from build123d import *

# Parameters (mm, degrees)
F0_R     = 2.867556
F1_DEPTH = 20
F3_DEPTH = 5


with BuildPart() as f1:
    # F0 (on Top) → F1 (new body)
    with BuildSketch(Plane.XY):
        Polygon((49.845867, -3.922955), (45, 0), (49.845867, 3.922955), (44.445975, 7.039551), (48.618496, 11.672268), (42.797543, 13.905765), (46.193977, 19.134172), (40.095294, 20.429572), (42.632008, 26.124928), (36.405765, 26.450336), (38.020298, 32.472402), (31.819805, 31.819805), (32.472402, 38.020298), (26.450336, 36.405765), (26.124928, 42.632008), (20.429572, 40.095294), (19.134172, 46.193977), (13.905765, 42.797543), (11.672268, 48.618496), (7.039551, 44.445975), (3.922955, 49.845867), (0, 45), (-3.922955, 49.845867), (-7.039551, 44.445975), (-11.672268, 48.618496), (-13.905765, 42.797543), (-19.134172, 46.193977), (-20.429572, 40.095294), (-26.124928, 42.632008), (-26.450336, 36.405765), (-32.472402, 38.020298), (-31.819805, 31.819805), (-38.020298, 32.472402), (-36.405765, 26.450336), (-42.632008, 26.124928), (-40.095294, 20.429572), (-46.193977, 19.134172), (-42.797543, 13.905765), (-48.618496, 11.672268), (-44.445975, 7.039551), (-49.845867, 3.922955), (-45, 0), (-49.845867, -3.922955), (-44.445975, -7.039551), (-48.618496, -11.672268), (-42.797543, -13.905765), (-46.193977, -19.134172), (-40.095294, -20.429572), (-42.632008, -26.124928), (-36.405765, -26.450336), (-38.020298, -32.472402), (-31.819805, -31.819805), (-32.472402, -38.020298), (-26.450336, -36.405765), (-26.124928, -42.632008), (-20.429572, -40.095294), (-19.134172, -46.193977), (-13.905765, -42.797543), (-11.672268, -48.618496), (-7.039551, -44.445975), (-3.922955, -49.845867), (0, -45), (3.922955, -49.845867), (7.039551, -44.445975), (11.672268, -48.618496), (13.905765, -42.797543), (19.134172, -46.193977), (20.429572, -40.095294), (26.124928, -42.632008), (26.450336, -36.405765), (32.472402, -38.020298), (31.819805, -31.819805), (38.020298, -32.472402), (36.405765, -26.450336), (42.632008, -26.124928), (40.095294, -20.429572), (46.193977, -19.134172), (42.797543, -13.905765), (48.618496, -11.672268), (44.445975, -7.039551), align=None)
        with Locations((-8.660254, -5)):
            Circle(F0_R, mode=Mode.SUBTRACT)
        with Locations((8.660254, -5)):
            Circle(F0_R, mode=Mode.SUBTRACT)
        with Locations((0, 10)):
            Circle(F0_R, mode=Mode.SUBTRACT)
    extrude(amount=F1_DEPTH)

    # F2 (on face) → F3 (cut)
    with BuildSketch(Plane.XY.offset(20)):
        Polygon((2.886751, 15), (-2.886751, 15), (-5.773503, 10), (-2.886751, 5), (2.886751, 5), (5.773503, 10), align=None)
        Polygon((-11.547005, 0), (-14.433757, -5), (-11.547005, -10), (-5.773503, -10), (-2.886751, -5), (-5.773503, 0), align=None)
        Polygon((5.773503, -10), (11.547005, -10), (14.433757, -5), (11.547005, 0), (5.773503, 0), (2.886751, -5), align=None)
    extrude(amount=-F3_DEPTH, mode=Mode.SUBTRACT)


solid = f1.part
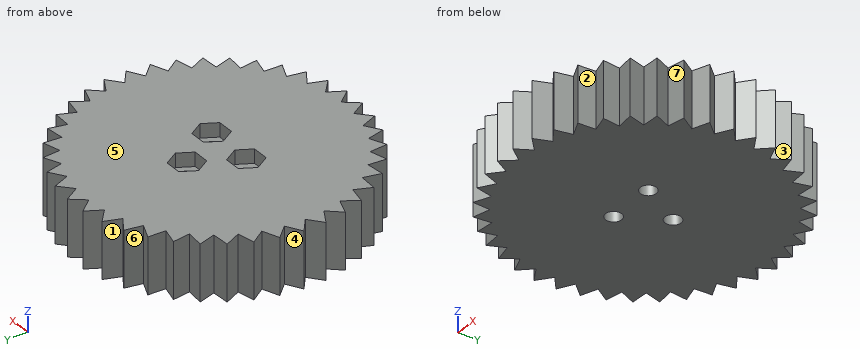
Part model, mm, in its own coordinate system. Face numbers are marked on the shaded views. A direction names the side the tool comes from. Coordinates: 2 decimals unless noted, no trailing zeros. Order: outer loops, then holes, each group sorted by start corner. A loop starts at its lowest first (then second) coordinate and runs counter-clockwise, first axis right, second up. Notation, with made-up numbers: M 51.25,8.25 L 72.25,8.25 A18 cw 72.25,25.25 Z; hole C 26,-24 d5. An arc over 180 degrees is marked long. One line per question, with ' | ' between items.
Q1. Drill centre lines: line 1 (X direction, y = -5, z = 4); line 2 (X direction, y = -6.5, z = 1.5); line 3 (Y direction, x = 0, z = 10.5). Where is each one in solid material? Low to high.
A:
line 1: x = -47.98 to -11.53, -5.79 to 5.79, 11.53 to 47.98 | line 2: x = -45.38 to -11.1, -6.22 to 6.22, 11.1 to 45.38 | line 3: y = -45 to 7.13, 12.87 to 45
Q2. Two-plate mould, pull along X, no slides. Class the marked faces 5, 6 and 7: +X half, -X half, draft (parallel to the pull), parting line (faces both ways), or undercut.
A:
face 5: draft | face 6: undercut | face 7: +X half
Q3. Slice it at C-C (x = -9). Give the cut face in (y, z), and give its area (3 significant figures).
A:
outline: M -46.21,0 L -7.85,0 L -7.85,15 L -10,15 L -10,20 L -46.21,20 Z; M -2.15,0 L 46.21,0 L 46.21,20 L 0,20 L 0,15 L -2.15,15 Z | area: 1,710 mm^2
Q4. Pin check, flat tips, straight feed: P1, Ø3, axis at x = -11, y = -4.5, coming from the +Z side; P2, Ø5.5, axis at x = -8, z = 17, coming from the -Y side; P3, Ø4, axis at x = 9.5, z = 17.5, coming from the -Y side; P4, Ø5, axis at x = 0, y = 10, coming from the -Z side. Stop position of each tip, or through.
A:
P1: stops at z = 15 | P2: stops at y = -47.79 | P3: stops at y = -48.46 | P4: passes through
Q5. 3-axis set-ups, long thin cutter, end or side, ignore diameter. For the marked faces 1, 2, 3 and 4: which of +Z, -Z, +X, -X, +Y, -Y reach the whole face in a straight line?
A:
face 1: +Z, -Z, +Y | face 2: +Z, -Z, -Y | face 3: +Z, -Z, +X | face 4: +Z, -Z, -X
Q6. Slice it at B-B (z = 8.5). Count the separate pieces of the cut face and the enclosed holes in it, and give its area (3 significant figures).
A:
separate pieces: 1 | enclosed holes: 3 | area: 6,980 mm^2
Q7. Slice it at D-D (y = 34). Give the cut face in (x, z).
A:
outline: M -32.05,0 L 32.05,0 L 32.05,20 L -32.05,20 Z
Q8. Slice it at A-A (x = 1.5). Give the cut face in (y, z).
A:
outline: M -46.85,0 L 7.56,0 L 7.56,15 L 5,15 L 5,20 L -46.85,20 Z; M 12.44,0 L 46.85,0 L 46.85,20 L 15,20 L 15,15 L 12.44,15 Z
